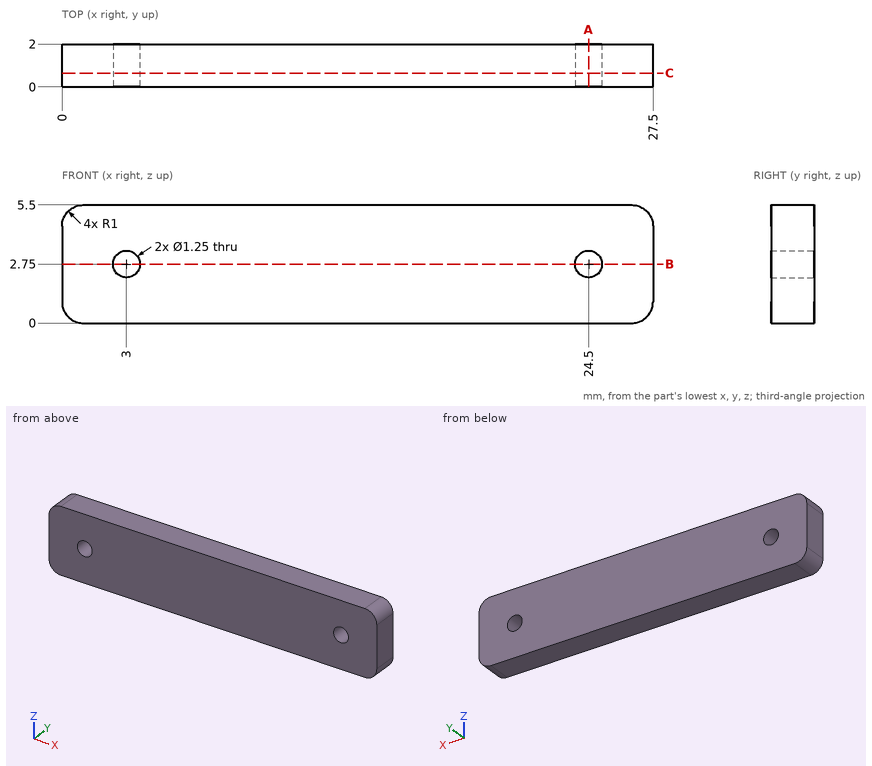
Geometry: see drawing. Coordinates: mm, zero at the bounding-box minimum. Coordinates: 2 decimals unless noted, no trailing zeros. Write each loop counter-clockwise with the first axis right and the second up, starting at its lowest first coordinate (ties: lowest second). Pieces come first, ordered by that corner, then holes.
1) Section B-B on z = 2.75. Output: boundary loops of the cut face in (x, y) (3 decimals).
2) Material intervals for line 1 along X through (y, z) = (0.8, 2.75) (3 decimals); line 2 along Z through (x, y) = (24.5, 1.4) (3 decimals); line 3 along X through (y, z) = (0.25, 2.3), sorted ascending.
3) Pin query (flat end, axial travel): pin 1 Ø1 at (x, y) = (21.5, 1.5) entering from -Z; pin 2 Ø1 at (x, z) = (24.5, 2.75) entering from +Y. Return the tip coordinate at first contact, or that it passes through.
4) Section C-C on y = 0.65. Output: boundary loops of the cut face in (x, z) (3 decimals).
5) Section A-A on x = 24.5. Output: boundary loops of the cut face in (y, z) (3 decimals).
Check result:
1. outline: (0, 0) - (2.375, 0) - (2.375, 2) - (0, 2) - close; (3.625, 0) - (23.875, 0) - (23.875, 2) - (3.625, 2) - close; (25.125, 0) - (27.5, 0) - (27.5, 2) - (25.125, 2) - close
2. line 1: x = 0 to 2.375, 3.625 to 23.875, 25.125 to 27.5
2. line 2: z = 0 to 2.125, 3.375 to 5.5
2. line 3: x = 0 to 2.57, 3.43 to 24.07, 24.93 to 27.5
3. pin 1: stops at z = 0
3. pin 2: passes through
4. outline: (0, 1) arc R1 ccw to (1, 0) - (26.5, 0) arc R1 ccw to (27.5, 1) - (27.5, 4.5) arc R1 ccw to (26.5, 5.5) - (1, 5.5) arc R1 ccw to (0, 4.5) - close; hole circle Ø1.25 at (3, 2.75); hole circle Ø1.25 at (24.5, 2.75)
5. outline: (0, 0) - (2, 0) - (2, 2.125) - (0, 2.125) - close; (0, 3.375) - (2, 3.375) - (2, 5.5) - (0, 5.5) - close
